Can you work these out from the model? Positions are in its coordinate system, mm. Coordinates: 2 decimals unless noted, no trailing zeros. Order: outer loops, then holes, each group sorted by start corner. A loop starts at its lowest first (then second) coordinate and runs counter-clockwise, first axis right, second up. Notation, with made-up numbers: (14.5, 20.5) -> (67.5, 20.5) arc R23 cw to (67.5, 32.5) -> close; hole circle Ø6 at (-23, 1). An arc over 180 degrees is marked (long way). Answer as CSV lines item,"result".
from build123d import *

# Parameters (mm, degrees)
BOX002_W         = 10
BOX002_H         = 10
BOX002_DEPTH     = 10
ARRAY001_X_COUNT = 5
ARRAY001_X_PITCH = 12
ARRAY001_Y_COUNT = 5
ARRAY001_Y_PITCH = 12
BOX003_W         = 62
BOX003_H         = 62
BOX003_DEPTH     = 3


with BuildPart() as array001:
    # Box002 → Box002 (new body)
    with BuildSketch(Plane.XY):
        with Locations((5, 5)):
            Rectangle(BOX002_W, BOX002_H)
    extrude(amount=BOX002_DEPTH)

    # Array001 X: Array001 ×5


with BuildPart() as array001_1:
    add(array001.part)
    with Locations(*[(i * ARRAY001_X_PITCH, 0, 0) for i in range(1, ARRAY001_X_COUNT)]):
        add(array001.part)

    # Array001 Y: Array001 ×5


with BuildPart() as array001_2:
    add(array001_1.part)
    with Locations(*[(0, i * ARRAY001_Y_PITCH, 0) for i in range(1, ARRAY001_Y_COUNT)]):
        add(array001_1.part)


with BuildPart() as cut001:
    # Box003 → Box003 (new body)
    with BuildSketch(Plane(origin=(-2, -2, 3), x_dir=(1, 0, 0), z_dir=(0, 0, 1))):
        with Locations((31, 31)):
            Rectangle(BOX003_W, BOX003_H)
    extrude(amount=BOX003_DEPTH)

    # Cut001: cut Array001
    add(array001_2.part, mode=Mode.SUBTRACT)


solid = cut001.part
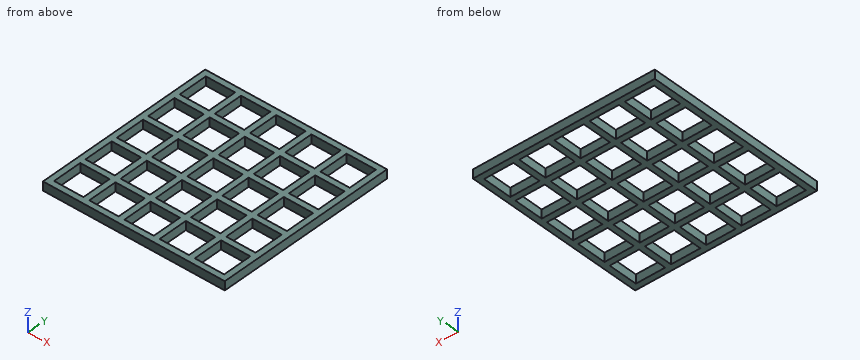
Q1. Imagine slicing it at A-A (x = 32.5). List the corners of the cut face in (y, z) for me, and give its area (3 significant figures).
Solution:
outline,"(-2, 3) -> (0, 3) -> (0, 6) -> (-2, 6) -> close; (10, 3) -> (12, 3) -> (12, 6) -> (10, 6) -> close; (22, 3) -> (24, 3) -> (24, 6) -> (22, 6) -> close; (34, 3) -> (36, 3) -> (36, 6) -> (34, 6) -> close; (46, 3) -> (48, 3) -> (48, 6) -> (46, 6) -> close; (58, 3) -> (60, 3) -> (60, 6) -> (58, 6) -> close"
area,"36.0 mm2"
Q2. For P1, Ø1.5, axis at x = 17, y = 33.5, coming from the +Z side, with a flat end and sliding along its axis, tell me the tip position at first contact or that it passes through.
Solution:
P1,"z = 6"
Q3. Imagine slicing it at C-C (z = 4.35). Give the number of separate pieces and of enclosed holes in the cut face, and give its area (3 significant figures).
Solution:
separate pieces,"1"
enclosed holes,"25"
area,"1,340 mm2"
Q4. If I drill on line 1 (Y direction, x = 17, z = 5.45), over which ranges is the centre line in solid material (lowest first)?
Solution:
line 1,"-2 to 0, 10 to 12, 22 to 24, 34 to 36, 46 to 48, 58 to 60"
